The model under review builds one solid part; all positions refer to its coordinate system, in mm. A direction names the side the tool comes from. Coordinates: 2 decimals unless noted, no trailing zeros. Order: outer loops, then holes, each group sorted by start corner. A loop starts at its lowest first (then second) coordinate and runs counter-clockwise, first axis right, second up. Notation, with made-up numbers: (-29, -32) - (-17, -32) arc R13 cw to (-17, -9) - close; hole circle Ø10 at (-21, -24.5). An arc over 180 degrees is marked (long way). Answer in a Markdown table with one row per item.
```python
from build123d import *

# Parameters (mm, degrees)
SKETCH_1_R               = 6.25
EXTRUDE_627_DEPTH        = 8
SKETCH_2_R               = 8
CUT_EXTRUDE_911_DEPTH    = 4
SKETCH_3_R               = 1.7
CUT_EXTRUDE_3_DEPTH      = 60.372950698
PATTERN_CIRCULAR_1_COUNT = 6
SKETCH_4_R               = 47.5
SKETCH_4_R_2             = 23.25
CUT_EXTRUDE_3_2_DEPTH    = 4
FILLET_1_R               = 10
FILLET_2_R               = 24
FILLET_3_R               = 4
SKETCH_5_R               = 3
CUT_EXTRUDE_2981_DEPTH   = 57.344747555
PATTERN_CIRCULAR_2_COUNT = 3


# Some blends are built 0.0001 mm under size
with BuildPart() as part:
    # Эскиз1 → Extrude 627 (new body)
    with BuildSketch(Plane(origin=(0, 0, 0), x_dir=(1, 0, 0), z_dir=(0, 1, 0))):
        Polygon((-17, 9.814954576), (-17, 40), (17, 40), (17, 9.814954576), (43.141016151, -5.277568136), (26.141016151, -34.722431864), (0, -19.629909152), (-26.141016151, -34.722431864), (-43.141016151, -5.277568136), align=None)
        with Locations(Location((0, 0, 0), (0, 0, 270))):
            Circle(SKETCH_1_R, mode=Mode.SUBTRACT)
    extrude(amount=EXTRUDE_627_DEPTH)

    # Эскиз2 → Cut-Extrude 911 (cut)
    with BuildSketch(Plane(origin=(0, 0, 0), x_dir=(1, 0, 0), z_dir=(0, 1, 0))):
        with Locations(Location((0, 0, 0), (0, 0, 270))):
            Circle(SKETCH_2_R)
    extrude(amount=CUT_EXTRUDE_911_DEPTH, mode=Mode.SUBTRACT)

    # Эскиз3 → Cut-Extrude 3 (cut, through all)
    with BuildSketch(Plane(origin=(0, 8, 0), x_dir=(1, 0, 0), z_dir=(0, 1, 0))):
        with Locations(Location((0, 12.5, 0), (0, 0, 270))):
            Circle(SKETCH_3_R)
    cut_extrude_3 = extrude(amount=-CUT_EXTRUDE_3_DEPTH, mode=Mode.SUBTRACT)

    # Круговой массив1: Cut-Extrude 3 ×6 about axis
    pattern_circular_1_axis = Axis((0, 0, 0), (0, 1, 0))
    for i in range(1, PATTERN_CIRCULAR_1_COUNT):
        add(cut_extrude_3.rotate(pattern_circular_1_axis, i * 360 / PATTERN_CIRCULAR_1_COUNT), mode=Mode.SUBTRACT)

    # Эскиз4 → Cut-Extrude 3 2 (cut)
    with BuildSketch(Plane.XZ.offset(-8)):
        Circle(SKETCH_4_R)
        Circle(SKETCH_4_R_2, mode=Mode.SUBTRACT)
    extrude(amount=CUT_EXTRUDE_3_2_DEPTH, mode=Mode.SUBTRACT)

    # Скругление1
    fillet_1_edges = [part.edges().sort_by_distance(p)[0] for p in [
        (-17, 2, -40),
        (17, 2, -40),
        (43.141016151, 2, 5.277568136),
        (26.141016151, 2, 34.722431864),
        (-26.141016151, 2, 34.722431864),
        (-43.141016151, 2, 5.277568136),
    ]]
    fillet(fillet_1_edges, radius=FILLET_1_R)

    # Скругление2
    # the kernel refuses this fillet: 24 mm, written as the material it adds along each edge
    with BuildSketch(Plane(origin=(17, 0, -9.814954576), x_dir=(0, 0, -1), z_dir=(0, 1, 0))) as fillet_2_piece_1_section:
        with BuildLine():
            CenterArc((FILLET_2_R * 0.57735026919, -FILLET_2_R), FILLET_2_R, 90, 60)
            Line((-FILLET_2_R * 0.288675134595, -FILLET_2_R * 0.5), (0, 0))
            Line((0, 0), (FILLET_2_R * 0.57735026919, 0))
        make_face()
    fillet_2_piece_1 = extrude(amount=8, mode=Mode.PRIVATE)
    fillet_2_piece_1 = split(fillet_2_piece_1, bisect_by=Plane(origin=(20.179222724, 4, -11.650479672), z_dir=(0, -1, 0)), keep=Keep.TOP, mode=Mode.PRIVATE)
    fillet_2_piece_1 = fillet_2_piece_1 - Plane(origin=(0, 2, 0), x_dir=(1, 0, 0), z_dir=(0, 1, 0)) * Cylinder(23.25, 72, mode=Mode.PRIVATE)
    add(fillet_2_piece_1)
    with BuildSketch(Plane(origin=(17, 0, -9.814954576), x_dir=(0, 0, -1), z_dir=(0, 1, 0))) as fillet_2_piece_2_section:
        with BuildLine():
            CenterArc((FILLET_2_R * 0.57735026919, -FILLET_2_R), FILLET_2_R, 90, 60)
            Line((-FILLET_2_R * 0.288675134595, -FILLET_2_R * 0.5), (0, 0))
            Line((0, 0), (FILLET_2_R * 0.57735026919, 0))
        make_face()
    fillet_2_piece_2 = extrude(amount=8, mode=Mode.PRIVATE)
    fillet_2_piece_2 = split(fillet_2_piece_2, bisect_by=Plane(origin=(18.777250195, 4, -10.841050455), z_dir=(0, -1, 0)), keep=Keep.TOP, mode=Mode.PRIVATE)
    fillet_2_piece_2 = fillet_2_piece_2 & Plane(origin=(0, 2, 0), x_dir=(1, 0, 0), z_dir=(0, 1, 0)) * Cylinder(23.25, 72, mode=Mode.PRIVATE)
    add(fillet_2_piece_2)
    with BuildSketch(Plane(origin=(17, 0, -9.814954576), x_dir=(0, 0, -1), z_dir=(0, 1, 0))) as fillet_2_piece_3_section:
        with BuildLine():
            CenterArc((FILLET_2_R * 0.57735026919, -FILLET_2_R), FILLET_2_R, 90, 60)
            Line((-FILLET_2_R * 0.288675134595, -FILLET_2_R * 0.5), (0, 0))
            Line((0, 0), (FILLET_2_R * 0.57735026919, 0))
        make_face()
    fillet_2_piece_3 = extrude(amount=8, mode=Mode.PRIVATE)
    fillet_2_piece_3 = split(fillet_2_piece_3, bisect_by=Plane(origin=(18.777250195, 4, -10.841050455), z_dir=(0, 1, 0)), keep=Keep.TOP, mode=Mode.PRIVATE)
    fillet_2_piece_3 = fillet_2_piece_3 & Plane(origin=(0, 6, 0), x_dir=(1, 0, 0), z_dir=(0, 1, 0)) * Cylinder(23.25, 72, mode=Mode.PRIVATE)
    add(fillet_2_piece_3)
    with BuildSketch(Plane(origin=(-17, 0, -9.814954576), x_dir=(0, 0, -1), z_dir=(0, 1, 0))) as fillet_2_piece_4_section:
        with BuildLine():
            CenterArc((FILLET_2_R * 0.57735026919, FILLET_2_R), FILLET_2_R, 210, 60)
            Line((-FILLET_2_R * 0.288675134595, FILLET_2_R * 0.5), (0, 0))
            Line((0, 0), (FILLET_2_R * 0.57735026919, 0))
        make_face()
    fillet_2_piece_4 = extrude(amount=8, mode=Mode.PRIVATE)
    fillet_2_piece_4 = split(fillet_2_piece_4, bisect_by=Plane(origin=(-20.179222724, 4, -11.650479672), z_dir=(0, -1, 0)), keep=Keep.TOP, mode=Mode.PRIVATE)
    fillet_2_piece_4 = fillet_2_piece_4 - Plane(origin=(0, 2, 0), x_dir=(1, 0, 0), z_dir=(0, 1, 0)) * Cylinder(23.25, 72, mode=Mode.PRIVATE)
    add(fillet_2_piece_4)
    with BuildSketch(Plane(origin=(-17, 0, -9.814954576), x_dir=(0, 0, -1), z_dir=(0, 1, 0))) as fillet_2_piece_5_section:
        with BuildLine():
            CenterArc((FILLET_2_R * 0.57735026919, FILLET_2_R), FILLET_2_R, 210, 60)
            Line((-FILLET_2_R * 0.288675134595, FILLET_2_R * 0.5), (0, 0))
            Line((0, 0), (FILLET_2_R * 0.57735026919, 0))
        make_face()
    fillet_2_piece_5 = extrude(amount=8, mode=Mode.PRIVATE)
    fillet_2_piece_5 = split(fillet_2_piece_5, bisect_by=Plane(origin=(-18.777250195, 4, -10.841050455), z_dir=(0, -1, 0)), keep=Keep.TOP, mode=Mode.PRIVATE)
    fillet_2_piece_5 = fillet_2_piece_5 & Plane(origin=(0, 2, 0), x_dir=(1, 0, 0), z_dir=(0, 1, 0)) * Cylinder(23.25, 72, mode=Mode.PRIVATE)
    add(fillet_2_piece_5)
    with BuildSketch(Plane(origin=(-17, 0, -9.814954576), x_dir=(0, 0, -1), z_dir=(0, 1, 0))) as fillet_2_piece_6_section:
        with BuildLine():
            CenterArc((FILLET_2_R * 0.57735026919, FILLET_2_R), FILLET_2_R, 210, 60)
            Line((-FILLET_2_R * 0.288675134595, FILLET_2_R * 0.5), (0, 0))
            Line((0, 0), (FILLET_2_R * 0.57735026919, 0))
        make_face()
    fillet_2_piece_6 = extrude(amount=8, mode=Mode.PRIVATE)
    fillet_2_piece_6 = split(fillet_2_piece_6, bisect_by=Plane(origin=(-18.777250195, 4, -10.841050455), z_dir=(0, 1, 0)), keep=Keep.TOP, mode=Mode.PRIVATE)
    fillet_2_piece_6 = fillet_2_piece_6 & Plane(origin=(0, 6, 0), x_dir=(1, 0, 0), z_dir=(0, 1, 0)) * Cylinder(23.25, 72, mode=Mode.PRIVATE)
    add(fillet_2_piece_6)
    with BuildSketch(Plane(origin=(0, 0, 19.629909152), x_dir=(-0.8660254037844384, 0, 0.5000000000000003), z_dir=(0, 1, 0))) as fillet_2_piece_7_section:
        with BuildLine():
            CenterArc((FILLET_2_R * 0.57735026919, FILLET_2_R), FILLET_2_R, 210, 60)
            Line((-FILLET_2_R * 0.288675134595, FILLET_2_R * 0.5), (0, 0))
            Line((0, 0), (FILLET_2_R * 0.57735026919, 0))
        make_face()
    fillet_2_piece_7 = extrude(amount=8, mode=Mode.PRIVATE)
    fillet_2_piece_7 = split(fillet_2_piece_7, bisect_by=Plane(origin=(0, 4, 23.300959344), z_dir=(0, -1, 0)), keep=Keep.TOP, mode=Mode.PRIVATE)
    fillet_2_piece_7 = fillet_2_piece_7 - Plane(origin=(0, 2, 0), x_dir=(1, 0, 0), z_dir=(0, 1, 0)) * Cylinder(23.25, 72, mode=Mode.PRIVATE)
    add(fillet_2_piece_7)
    with BuildSketch(Plane(origin=(0, 0, 19.629909152), x_dir=(-0.8660254037844384, 0, 0.5000000000000003), z_dir=(0, 1, 0))) as fillet_2_piece_8_section:
        with BuildLine():
            CenterArc((FILLET_2_R * 0.57735026919, FILLET_2_R), FILLET_2_R, 210, 60)
            Line((-FILLET_2_R * 0.288675134595, FILLET_2_R * 0.5), (0, 0))
            Line((0, 0), (FILLET_2_R * 0.57735026919, 0))
        make_face()
    fillet_2_piece_8 = extrude(amount=8, mode=Mode.PRIVATE)
    fillet_2_piece_8 = split(fillet_2_piece_8, bisect_by=Plane(origin=(0, 4, 21.68210091), z_dir=(0, -1, 0)), keep=Keep.TOP, mode=Mode.PRIVATE)
    fillet_2_piece_8 = fillet_2_piece_8 & Plane(origin=(0, 2, 0), x_dir=(1, 0, 0), z_dir=(0, 1, 0)) * Cylinder(23.25, 72, mode=Mode.PRIVATE)
    add(fillet_2_piece_8)
    with BuildSketch(Plane(origin=(0, 0, 19.629909152), x_dir=(-0.8660254037844384, 0, 0.5000000000000003), z_dir=(0, 1, 0))) as fillet_2_piece_9_section:
        with BuildLine():
            CenterArc((FILLET_2_R * 0.57735026919, FILLET_2_R), FILLET_2_R, 210, 60)
            Line((-FILLET_2_R * 0.288675134595, FILLET_2_R * 0.5), (0, 0))
            Line((0, 0), (FILLET_2_R * 0.57735026919, 0))
        make_face()
    fillet_2_piece_9 = extrude(amount=8, mode=Mode.PRIVATE)
    fillet_2_piece_9 = split(fillet_2_piece_9, bisect_by=Plane(origin=(0, 4, 21.68210091), z_dir=(0, 1, 0)), keep=Keep.TOP, mode=Mode.PRIVATE)
    fillet_2_piece_9 = fillet_2_piece_9 & Plane(origin=(0, 6, 0), x_dir=(1, 0, 0), z_dir=(0, 1, 0)) * Cylinder(23.25, 72, mode=Mode.PRIVATE)
    add(fillet_2_piece_9)

    # Скругление3
    fillet_3_edges = [part.edges().sort_by_distance(p)[0] for p in [
        (-5.23578811, 8, -22.652792827),
    ]]
    fillet(fillet_3_edges, radius=FILLET_3_R - 0.0001)  # a hair under: the kernel refuses the full size

    # Эскиз5 → Cut-Extrude 2981 (cut, through all)
    with BuildSketch(Plane(origin=(0, 4, 0), x_dir=(-1, 0, 0), z_dir=(0, 1, 0))):
        with Locations(Location((-9.25, -31.898395826, 0), (0, 0, 90))):
            Circle(SKETCH_5_R)
        with Locations(Location((-32.249821125, 7.938462928, 0), (0, 0, 90))):
            Circle(SKETCH_5_R)
    cut_extrude_2981 = extrude(amount=-CUT_EXTRUDE_2981_DEPTH, mode=Mode.SUBTRACT)

    # Круговой массив2: Cut-Extrude 2981 ×3 about axis
    pattern_circular_2_axis = Axis((0, 0, 0), (0, 1, 0))
    for i in range(1, PATTERN_CIRCULAR_2_COUNT):
        add(cut_extrude_2981.rotate(pattern_circular_2_axis, i * 360 / PATTERN_CIRCULAR_2_COUNT), mode=Mode.SUBTRACT)


solid = part.part
```
Item 1: We need section A-A, the plane x = 0. State how many separate pieces and enclosed holes the cut face has, then the cut area to 3 significant figures.
Check values:
| item | result |
|---|---|
| separate pieces | 4 |
| enclosed holes | 0 |
| area | 264 mm^2 |
Item 2: Tool access review of faces 1 (the face through (-8.349, 2.028, -29.037)), 2 (the face through (17, 2, -27)), 3 (the face through (-14.702, 1.972, 28.118)), 4 (the face through (-17, 2, -27)), 5 (the face through (39.17, 2.03, 6.46)): name each direction out of +Z, -Z, +X, -X, +Y, -Y from which nothing blocks a thin tool from reaching the whole face with its end or side.
Check values:
| item | result |
|---|---|
| face 1 | +Y, -Y |
| face 2 | -Z, +X, +Y, -Y |
| face 3 | +Z, +Y, -Y |
| face 4 | -Z, -X, +Y, -Y |
| face 5 | +X, +Y, -Y |
Item 3: We need section B-B, the plane z = -31.5. Write out the cut boundary in (x, y), then the cut area to 3 significant figures.
Check values:
| item | result |
|---|---|
| outline | (-16.89, 0) - (-12.22, 0) - (-12.22, 4) - (-16.89, 4) - close; (-6.28, 0) - (6.28, 0) - (6.28, 4) - (-6.28, 4) - close; (12.22, 0) - (16.89, 0) - (16.89, 4) - (12.22, 4) - close |
| area | 87.5 mm^2 |
Item 4: Mouldability with a two-part tool opening along Z and no side actions: class faces 6 (the face through (14.15, 2.03, -36.99)), 7 (the face through (-1.7, 8, 6.2)), 8 (the face through (-9.14, 4.06, 6.03)) as +Z half, -Z half, draft (parallel to the pull), parting line (faces both ways), or undercut.
Check values:
| item | result |
|---|---|
| face 6 | -Z half |
| face 7 | draft |
| face 8 | undercut |
Item 5: Clearance check with flat-ended pins moving along their axes: pin 1 Ø9.5 at (x, z) = (-23, 23.96) entering from +Y; pin 2 Ø2 at (x, y) = (-3.5, 7) entering from -Z; pin 3 Ø3 at (y, z) = (2.5, -26) entering from +X. State where each tip first meets the part, or that it passes through.
Check values:
| item | result |
|---|---|
| pin 1 | y = 4 |
| pin 2 | z = -22.46 |
| pin 3 | x = 17 |
Item 6: We need section C-C, the plane y = 5. Write out the cut boundary in (x, z).
Check values:
| item | result |
|---|---|
| outline | circle Ø46.25 at (0, 0); hole circle Ø3.4 at (-10.83, -6.25); hole circle Ø3.4 at (-10.83, 6.25); hole circle Ø12.5 at (0, 0); hole circle Ø3.4 at (0, -12.5); hole circle Ø3.4 at (0, 12.5); hole circle Ø3.4 at (10.83, -6.25); hole circle Ø3.4 at (10.83, 6.25) |
Item 7: To check wall thickness, follow line 1 (Z direction, x = -1, y = 2.5); line 2 (Y direction, x = -19.5, z = 13.5); line 3 (X direction, y = 0.5, z = -3). State the ranges of each line that lie inside material, in increasing order. Write a range as from..to.
Check values:
| item | result |
|---|---|
| line 1 | -40..-13.87, -11.13..-7.94, 7.94..11.13, 13.87..23.36 |
| line 2 | 0..4 |
| line 3 | -28.81..-7.42, 7.42..28.81 |
